Design review of the part built by this model. Coordinates are the model's own, in mm. Face numbers are marked on the shaded views. A direction names the side the tool comes from. Give positions to 0.01 mm unless a question says otherwise; leave off trailing zeros. Loops run counter-clockwise (first coordinate to the right, second up) from the corner with the lowest first, then second, coordinate; pieces in that order, holes last. Notation, with made-up numbers: (4, -28.5) -> (62, -28.5) arc R24 cw to (62, -7.5) -> close; hole circle Ø3 at (70.5, 49). An arc over 180 degrees is marked (long way). Use a Markdown table: item, result. Add a question column.
1. Add section B-B (x = 1). State the section outline as (y, z) points, and give its area (3 significant figures).
2. Add section A-A (z = 4). State the section outline as (x, y) points.
3. For pin 1 Ø9 at (x, y) = (0, 100) entering from +Z; pin 2 Ø6 at (x, z) = (-19.5, 2.5) entering from -Y; pin 3 Ø3 at (y, z) = (-3, 1.5) entering from +X; pin 4 Ø4 at (x, z) = (8.5, -25.5) entering from -Y, all flat-tipped, find the tip position at first contact; note any pin that passes through.
4. Draft analysis for pull direction Y (two halves, no side actions). For the marked faces 1, 2 and 3, state which applies: pulls with the +Y half, pulls with the -Y half, needs draft (parallel to the pull), parting line crosses it, or undercut.
5. Add section D-D (y = 106). State the section outline as (x, z) points.
6. For the marked faces 4 and 5, list the 3-axis set-ups (+Z, -Z, +X, -X, +Y, -Y) from which the entire face can be reached by the end or side of a thin tool; tool diameter is ignored.
7. To check wall thickness, follow line 1 (Y direction, x = 0, z = -34.75); line 2 (Z direction, x = 3.5, y = 16.5); line 3 (X direction, y = -1, z = -32.5). State the ranges of each line that lie inside material, in increasing order.
8. Add section C-C (x = -26). State the section outline as (y, z) points, and give its area (3 significant figures).
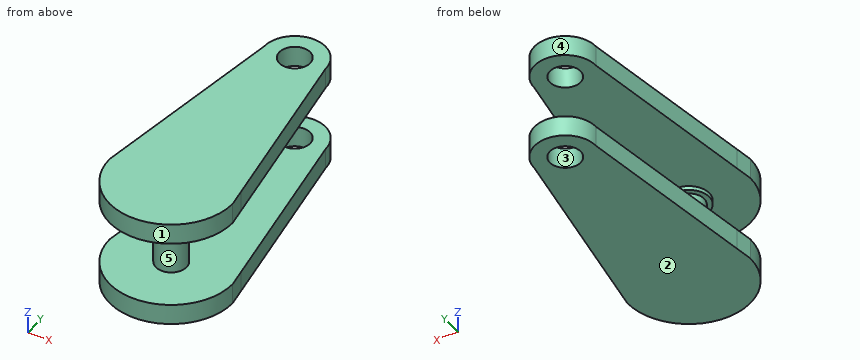
```python
from build123d import *

# Parameters (mm, degrees)
SKETCH1_R           = 7.5
SKETCH1_R_2         = 5
BOSS_EXTRUDE4_DEPTH = 10
BOSS_EXTRUDE5_START = -52
SKETCH6_R           = 7.5
BOSS_EXTRUDE5_DEPTH = 52
BOSS_EXTRUDE7_START = 2
SKETCH8_R           = 10
SKETCH8_R_2         = 7.5
BOSS_EXTRUDE7_DEPTH = 2
SKETCH10_R          = 7.5
CUT_EXTRUDE2_DEPTH  = 130.726635661


with BuildPart() as part:
    # Sketch1 → Boss-Extrude4 (new body)
    with BuildSketch(Plane.XY):
        with BuildLine():
            ThreePointArc((15, 100), (0, 115), (-15, 100))
            Line((-15, 100), (-28.679706601, 8.80195599))
            Line((-28.679706601, 8.80195599), (-30, 0))
            ThreePointArc((-30, 0), (0, -30), (30, 0))
            Line((30, 0), (28.679706601, 8.80195599))
            Line((28.679706601, 8.80195599), (15, 100))
        make_face()
        Circle(SKETCH1_R, mode=Mode.SUBTRACT)
        with Locations((0, 100)):
            Circle(SKETCH1_R_2, mode=Mode.SUBTRACT)
    boss_extrude4 = extrude(amount=BOSS_EXTRUDE4_DEPTH)

    # Sketch6 → Boss-Extrude5 (add)
    with BuildSketch(Plane.XY.offset(10).offset(BOSS_EXTRUDE5_START)):
        Circle(SKETCH6_R)
    extrude(amount=BOSS_EXTRUDE5_DEPTH)

    # Mirror1: Boss-Extrude4 across plane
    add(boss_extrude4.mirror(Plane.XY.offset(-16)))

    # Sketch8 → Boss-Extrude7 (add)
    with BuildSketch(Plane(origin=(0, 0, 0), x_dir=(-1, 0, 0), z_dir=(0, 0, -1)).offset(BOSS_EXTRUDE7_START)):
        with Locations(Location((0, 0, 0), (0, 0, 180))):
            Circle(SKETCH8_R)
        with Locations(Location((0, 0, 0), (0, 0, 180))):
            Circle(SKETCH8_R_2, mode=Mode.SUBTRACT)
    extrude(amount=-BOSS_EXTRUDE7_DEPTH)

    # Sketch10 → Cut-Extrude2 (cut, through all)
    with BuildSketch(Plane(origin=(0, 0, -42), x_dir=(-1, 0, 0), z_dir=(0, 0, -1))):
        with Locations((0, 100)):
            Circle(SKETCH10_R)
    extrude(amount=-CUT_EXTRUDE2_DEPTH, mode=Mode.SUBTRACT)


solid = part.part
```
Taken from the geometry:
| question | item | result |
|---|---|---|
| 1 | outline | (-29.98, -42) -> (92.57, -42) -> (92.57, -32) -> (7.43, -32) -> (7.43, -2) -> (9.95, -2) -> (9.95, 0) -> (92.57, 0) -> (92.57, 10) -> (-29.98, 10) -> (-29.98, 0) -> (-9.95, 0) -> (-9.95, -2) -> (-7.43, -2) -> (-7.43, -32) -> (-29.98, -32) -> close; (107.43, -42) -> (114.97, -42) -> (114.97, -32) -> (107.43, -32) -> close; (107.43, 0) -> (114.97, 0) -> (114.97, 10) -> (107.43, 10) -> close |
| 1 | area | 3,090 mm^2 |
| 2 | outline | (-30, 0) arc R30 ccw to (30, 0) -> (15, 100) arc R15 ccw to (-15, 100) -> close; hole circle Ø15 at (0, 100) |
| 3 | pin 1 | passes through |
| 3 | pin 2 | stops at y = -25.05 |
| 3 | pin 3 | stops at x = 29.96 |
| 3 | pin 4 | stops at y = -3.74 |
| 4 | face 1 | pulls with the -Y half |
| 4 | face 2 | needs draft |
| 4 | face 3 | undercut |
| 5 | outline | (-13.75, -42) -> (-4.5, -42) -> (-4.5, -32) -> (-13.75, -32) -> close; (-13.75, 0) -> (-4.5, 0) -> (-4.5, 10) -> (-13.75, 10) -> close; (4.5, -42) -> (13.75, -42) -> (13.75, -32) -> (4.5, -32) -> close; (4.5, 0) -> (13.75, 0) -> (13.75, 10) -> (4.5, 10) -> close |
| 6 | face 4 | +Z, -Z, +Y |
| 6 | face 5 | none |
| 7 | line 1 | y = -30 to 92.5, 107.5 to 115 |
| 7 | line 2 | z = -42 to -32, 0 to 10 |
| 7 | line 3 | x = -29.98 to 29.98 |
| 8 | outline | (-14.97, -42) -> (26.67, -42) -> (26.67, -32) -> (-14.97, -32) -> close; (-14.97, 0) -> (26.67, 0) -> (26.67, 10) -> (-14.97, 10) -> close |
| 8 | area | 833 mm^2 |
